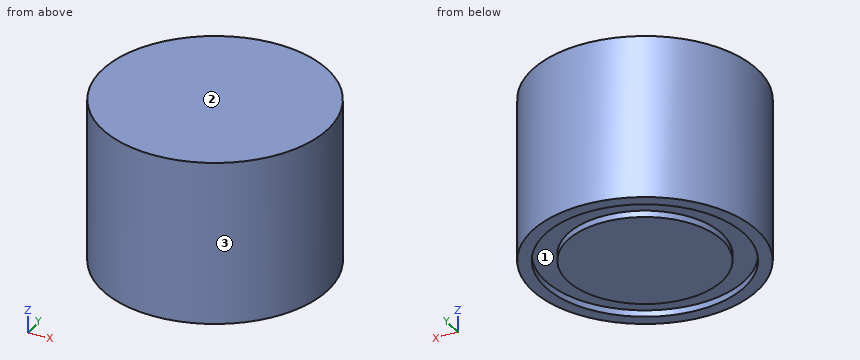
Autodesk Inventor part; units mm, degrees
ref_plane "XZ Plane" through (0, 0, 0) normal (0, 1, 0) x (-1, 0, 0)
ref_plane "XY Plane" through (0, 0, 0) normal (0, 0, 1) x (1, 0, 0)
sketch "Sketch1" plane through (0, 0, 0) normal (0, 0, 1) x (1, 0, 0)
  circle A0 centre (0, 0) radius 35
  dimension "d0" = 70
extrude "Extrusion1" add sketch "Sketch1" along normal blind 50.8
sketch "Sketch2" plane through (0, 0, 0) normal (0, 0, -1) x (-1, 0, 0)
  circle A0 centre (0, 0) radius 31
  circle A1 centre (0, 0) radius 24
  dimension "d3" = 62
  dimension "d4" = 48
extrude "Extrusion2" cut sketch "Sketch2" against normal blind 2
equation "\"d3\" = ringOuterDiam + ringDiamGap"
equation "\"d4\" = ringInnerDiam - ringDiamGap"
equation "\"ringOuterDiam\" = 60"
equation "\"ringInnerDiam\" = 50"
equation "\"ringThickness\" = 1.5"
equation "\"ringDiamGap\" = 2"
properties part number "MountV01"
Geometry check sheet. Reference: the model listing, model coordinates, mm. Face numbers are marked on the shaded views. Round coordinates to 2 decimals unless told otherwise and drop trailing zeros. Loops run counter-clockwise (first coordinate to the right, second up) from the corner with the lowest first, then second, coordinate; pieces in that order, holes last. Notation, with made-up numbers: (-3.5, 14.25) -> (14.5, 14.25) arc R25 ccw to (14.5, 27.25) -> close; hole circle Ø4 at (69.25, -11.5). An arc over 180 degrees is marked (long way). Answer as a JSON object with one key per item and string values. Group by question number.
Item 1: Cross-section at A-A, the plane z = 47. Record the cut outline in (x, y), plus the area to 3 significant figures.
Item 2: Cross-section at D-D, the plane y = -10. Record the cut outline in (x, z).
Item 3: Thickness scan on line 1 along Y through (x, z) = (0, 0.85); line 2 along Z through (x, y) = (-9, 23); line 3 along Y through (x, z) = (21, 41). Record the ranges inside material, lowest first.
Item 4: Cross-section at C-C, the plane y = 17. Record the cut outline in (x, z).
Item 5: Depth check by flat-ended pin: pin 1 Ø2 at (y, z) = (-8.5, 21) entering from +X; pin 2 Ø1 at (y, z) = (-14.5, 23.5) entering from +X; pin 3 Ø5 at (x, z) = (21, 7.5) entering from +Y. Enter the tip coordinate at first touch or a pass-through.
Item 6: Cross-section at B-B, the plane x = -28. Record the cut outline in (y, z).
Item 7: Release check for a two-part mould opening along X. For the marked faces 1, 2 and 3 record: pulls with the +X half, pulls with the -X half, needs draft (parallel to the pull), parting line crosses it, or undercut.
Determined:
{
 "1": {"outline": "circle Ø70 at (0, 0)", "area": "3,850 mm²"},
 "2": {"outline": "(-33.54, 0) -> (-29.34, 0) -> (-29.34, 2) -> (-21.82, 2) -> (-21.82, 0) -> (21.82, 0) -> (21.82, 2) -> (29.34, 2) -> (29.34, 0) -> (33.54, 0) -> (33.54, 50.8) -> (-33.54, 50.8) -> close"},
 "3": {"line 1": "y = -35 to -31, -24 to 24, 31 to 35", "line 2": "z = 2 to 50.8", "line 3": "y = -28 to 28"},
 "4": {"outline": "(-30.59, 0) -> (-25.92, 0) -> (-25.92, 2) -> (-16.94, 2) -> (-16.94, 0) -> (16.94, 0) -> (16.94, 2) -> (25.92, 2) -> (25.92, 0) -> (30.59, 0) -> (30.59, 50.8) -> (-30.59, 50.8) -> close"},
 "5": {"pin 1": "stops at x = 34.19", "pin 2": "stops at x = 32.08", "pin 3": "stops at y = 29.71"},
 "6": {"outline": "(-21, 0) -> (-13.3, 0) -> (-13.3, 2) -> (13.3, 2) -> (13.3, 0) -> (21, 0) -> (21, 50.8) -> (-21, 50.8) -> close"},
 "7": {"face 1": "undercut", "face 2": "needs draft", "face 3": "parting line crosses it"}
}
